Autodesk Inventor part; units mm, degrees
ref_plane "YZ Plane" through (0, 0, 0) normal (1, 0, 0) x (0, 1, 0)
ref_plane "XZ Plane" through (0, 0, 0) normal (0, 1, 0) x (-1, 0, 0)
ref_plane "XY Plane" through (0, 0, 0) normal (0, 0, 1) x (1, 0, 0)
sketch "Sketch1" plane through (0, 0, 0) normal (0, 0, 1) x (1, 0, 0)
  line L0 (0, 0) -> (50, 0)
  line L1 (50, 0) -> (50, 42.5)
  line L2 (50, 42.5) -> (0, 42.5)
  line L3 (0, 42.5) -> (0, 0)
  dimension "d0" = 50
  dimension "d1" = 42.5
extrude "Extrusion1" add sketch "Sketch1" along normal blind 7.5
sketch "Sketch2" plane through (0, 0, 0) normal (0, 0, -1) x (-1, 0, 0)
  line L0 (0, 42.5) -> (0, 0)
  line L1 (0, 35) -> (-7.5, 35)
  line L2 (-7.5, 35) -> (-7.5, 15)
  line L3 (-7.5, 15) -> (0, 15)
  line L4 (0, 15) -> (0, 35)
  line L5 (-50, 42.5) -> (0, 42.5)
  line L6 (0, 0) -> (-50, 0)
  point P0 (0, 15)
  dimension "d4" = 7.5
  dimension "d5" = 20
  dimension "d55" = 15
extrude "Extrusion2" add sketch "Sketch2" along normal blind 30
fillet "Fillet1" radius 10 2 edges at (3.75, 35, -30) (3.75, 15, -30)
sketch "Sketch3" plane through (7.5, 15, 0) normal (1, 0, 0) x (0, 0, -1)
  arc A0 (20, 0) -> (20, 20) centre (20, 10) ccw
  line L0 (30, 10) -> (20, 10) construction
  point P0 (0, -15)
hole "Hole1" at (7.5, 25, -20) direction (-1, 0, 0) diameter 4.8 end through all counterbore diameter 5.8 counterbore depth 4
chamfer "Chamfer1" distance 3 angle 45 2 edges at (3.75, 35, 0) (3.75, 15, 0)
sketch "Sketch6" plane through (0, 0, 7.5) normal (0, 0, 1) x (1, 0, 0)
  line L0 (50, 42.5) -> (0, 42.5)
  line L1 (25, 42.5) -> (25, -7.5) construction
  line L2 (12.5, 0) -> (12.5, 42.5)
  line L3 (12.5, 42.5) -> (37.5, 42.5)
  line L4 (37.5, 42.5) -> (37.5, 0)
  line L5 (37.5, 0) -> (12.5, 0)
  point P0 (0, 0)
  point P1 (45, 50)
  point P2 (5, 50)
  point P3 (0, 42.5)
  dimension "d43" = 50
  dimension "d44" = 42.5
  dimension "d45" = 25
  dimension "d46" = 42.5
  dimension "d47" = 12.5
extrude "Extrusion5" add sketch "Sketch6" along normal blind 100
sketch "Sketch10" plane through (12.5, 0, 7.5) normal (-1, 0, 0) x (0, 0, 1)
  line L0 (100, 42.5) -> (100, 0)
  line L1 (100, 35) -> (-7.5, 35)
  line L2 (-7.5, 35) -> (-7.5, 67.5)
  line L3 (-7.5, 67.5) -> (100, 67.5)
  line L4 (100, 67.5) -> (100, 35)
  line L5 (0, 42.5) -> (100, 42.5)
  point P0 (-7.5, 0)
  dimension "d66" = 107.5
  dimension "d67" = 32.5
  dimension "d68" = 7.5
extrude "Extrusion9" add sketch "Sketch10" along normal blind 25 and the other way blind 50
chamfer "Chamfer3" distance 25 distance2 20 1 edges at (25, 67.5, 0) measured on face at (19.1667, 57.6667, 0)
chamfer "Chamfer4" distance 25 distance2 20 1 edges at (25, 67.5, 107.5) measured on face at (20.8333, 56.6667, 107.5)
chamfer "Chamfer5" distance 10 angle 45 2 edges at (-12.5, 67.5, 53.75) (62.5, 67.5, 53.75)
chamfer "Chamfer6" distance 10 angle 45 1 edges at (25, 0, 107.5)
chamfer "Chamfer7" distance 5 angle 45 2 edges at (0, 0, 3.75) (50, 0, 3.75)
sketch "Sketch11" plane through (12.5, 0, 7.5) normal (-1, 0, 0) x (0, 0, 1)
  line L0 (0, 5) -> (0, 35)
  line L1 (0, 12.5) -> (100, 12.5) construction
  line L2 (0, 12.5) -> (100, 12.5) construction
  line L3 (0, 0) -> (90, 0)
  line L4 (100, 35) -> (0, 35)
  line L5 (27.5, 35) -> (27.5, 0) construction
  line L6 (90, 0) -> (90, 35) construction
  line L7 (100, 35) -> (100, 10)
  circle A0 centre (27.5, 12.5) radius 2.15
  circle A1 centre (90, 12.5) radius 2.15
  point P0 (-7.5, 0)
  dimension "d88" = 100
  dimension "d90" = 12.5
  dimension "d91" = 27.5
  dimension "d92" = 10
  dimension "d93" = 4.3
  dimension "d94" = 4.3
extrude "Extrusion10" cut sketch "Sketch11" against normal through all
properties part number "ES117_Head"
Model file for the job. Use its own axes, mm. A direction names the side the tool comes from. Give positions to 0.01 mm unless a question says otherwise; leave off trailing zeros. Order: outer loops, then holes, each group sorted by start corner. A loop starts at its lowest first (then second) coordinate and runs counter-clockwise, first axis right, second up. Notation, with made-up numbers: (69, -5.5) - (97, -5.5) arc R21 ccw to (97, 30.5) - close; hole circle Ø10 at (-23.75, -29). An arc over 180 degrees is marked (long way). Write item = value, one per line. Start each with the question number.
1. Cut at D-D, the plane x = -7.5. List the corners of the cut face in (y, z), and give its area (3 significant figures).
2. Cut at A-A, the plane z = 35. List the corners of the cut face in (x, y), and give its area (4 significant figures).
3. Probe line 1 along Z through (x, y) = (30, 12); line 2 along Y through (x, z) = (6.25, -20); line 3 along Z through (x, y) = (5.6, 25). List the from-to ranges inside material, lowest first.
4. Which spindle directions (+Z, -Z, +X, -X, +Y, -Y) get a long thin tool onto all of the face, cutting with end or side? Do faces 5 (the flat face through (7.5, 25, -15)), 6 (the flat face through (6, 18, 7.5)), 7 (the flat face through (4, 35, -11)), 8 (the cylindrical face through (5.472, 26.765, -17.699)). Say none if no direction does.
5. Cut at C-C, the plane y = 51. List the corners of the cut face in (x, z).
6. Cut at B-B, the plane x = 30. List the corners of the cut face in (y, z), and give its area (3 significant figures).
7. Two-plate mould, pull along Y, no slides. Class faces 1 (the flat face through (25, 67.5, 53)), 2 (the cylindrical face through (24.82, 13.15, 37.05)), 3 (the flat face through (48, 3, 4)), 4 (the flat face through (12.5, 17, 57)): pulls with the +Y half, pulls with the -Y half, needs draft (parallel to the pull), parting line crosses it, or undercut.
8. Drop flat-ended pins along their axis: P1, Ø4, axis at y = 21, z = 5.5, coming from the +X side; P2, Ø10, axis at x = 46.5, y = 15.5, coming from the +Z side; P3, Ø2.5, axis at y = 12.5, z = 35, coming from the -X side; P4, Ø12.5, axis at x = 55.5, z = 73.5, coming from the -Y side. Give the stop position or say it passes through.
Taken from the geometry:
q1.outline = (35, 0) - (42.5, 0) - (62.5, 16) - (62.5, 91.5) - (42.5, 107.5) - (35, 107.5) - close
q1.area = 2,640 mm²
q2.outline = (-12.5, 35) - (12.5, 35) - (12.5, 14.65) - (37.5, 14.65) - (37.5, 35) - (62.5, 35) - (62.5, 57.5) - (52.5, 67.5) - (-2.5, 67.5) - (-12.5, 57.5) - close; (12.5, 0) - (37.5, 0) - (37.5, 10.35) - (12.5, 10.35) - close
q2.area = 3,105 mm²
q3.line_1 = 0 to 32.91, 37.09 to 95.41, 99.59 to 107.5
q3.line_2 = 15 to 22.1, 27.9 to 35
q3.line_3 = -30 to -22.9, -17.1 to 7.5
q4.face_5 = -Z, +X, +Y, -Y
q4.face_6 = +Z, -X, -Y
q4.face_7 = -Z, +X, -X, +Y
q4.face_8 = +X
q5.outline = (-12.5, 6.8) - (62.5, 6.8) - (62.5, 100.7) - (-12.5, 100.7) - close
q6.outline = (0, 0) - (42.5, 0) - (67.5, 20) - (67.5, 87.5) - (42.5, 107.5) - (10, 107.5) - (0, 97.5) - close; hole circle Ø4.3 at (12.5, 35); hole circle Ø4.3 at (12.5, 97.5)
q6.area = 6,680 mm²
q7.face_1 = pulls with the +Y half
q7.face_2 = undercut
q7.face_3 = pulls with the -Y half
q7.face_4 = needs draft
q8.P1 = 50
q8.P2 = 7.5
q8.P3 = through
q8.P4 = 35
